The model under review builds one solid part; all positions refer to its coordinate system, in mm. A direction names the side the tool comes from. Round coordinates to 2 decimals unless told otherwise and drop trailing zeros. Order: outer loops, then holes, each group sorted by start corner. A loop starts at its lowest first (then second) coordinate and runs counter-clockwise, first axis right, second up.
from build123d import *

# Parameters (mm, degrees)
F0_W     = 127
F0_H     = 101.6
F1_DEPTH = 254
F2_SIZE  = 38.1
F3_W     = 50.8
F3_H     = 254
F4_DEPTH = 38.1
F5_SIZE  = 25.39999


# Not quite as in the source:
# - a fillet or chamfer is up to 0.001 mm smaller than in the source, because OpenCascade refuses the exact size


with BuildPart() as f1:
    # F0 (on Front) → F1 (new body)
    with BuildSketch(Plane.XZ):
        with Locations((63.5, 50.8)):
            Rectangle(F0_W, F0_H)
    extrude(amount=F1_DEPTH)

    # F2
    f2_edges = [f1.edges().sort_by_distance(p)[0] for p in [
        (127, -127, 101.6),
        (0, -127, 101.6),
    ]]
    chamfer(f2_edges, length=F2_SIZE)

    # F3 (on face) → F4 (join)
    with BuildSketch(Plane.XY.offset(101.6)):
        with Locations((63.5, -127)):
            Rectangle(F3_W, F3_H)
    extrude(amount=F4_DEPTH)

    # F5 (size 25.4 in the source; OpenCascade refuses exactly that, so slightly less here)
    f5_edges = [f1.edges().sort_by_distance(p)[0] for p in [
        (38.1, -127, 139.7),
        (88.9, -127, 139.7),
    ]]
    chamfer(f5_edges, length=F5_SIZE)


solid = f1.part
(1) Tool access review of faces 1 (the flat face through (38.1, -129, 108)), 2 (the flat face through (63, -125, 0)), 3 (the flat face through (88.9, -129, 108)): name each direction out of +Z, -Z, +X, -X, +Y, -Y from which nothing blocks a thin tool from reaching the whole face with its end or side.
(2) We need section B-B (x = 13.5). Give the boundary of the cut face in (y, z), and give its area (3 significant figures).
(3) Clearance check with flat-ended pins moving along their axes: P1, Ø5, axis at y = -109.5, z = 84.5, coming from the +X side; P2, Ø6, axis at x = 103.5, y = -132, coming from the +Z side; P3, Ø4, axis at y = -98, z = 114, coming from the +X side. State where each tip first meets the part, or that it passes through.
(4) To check wall thickness, follow L1, parallel to X at y = -172, z = 109; L2, parallel to X at y = -114, z = 131.5; L3, parallel to Z at x = 61, y = -84. State the ranges of each line that lie inside material, in increasing order.
(5) We need section C-C (z = 68.5). Give the boundary of the cut face in (x, y), and give its area (3 significant figures).
Verdict:
1. face 1: +Z, -X, +Y, -Y
1. face 2: -Z, +X, -X, +Y, -Y
1. face 3: +Z, +X, +Y, -Y
2. outline: (-254, 0) - (0, 0) - (0, 77) - (-254, 77) - close
2. area: 19,600 mm2
3. P1: stops at x = 108.5
3. P2: stops at z = 90
3. P3: stops at x = 88.9
4. L1: x = 38.1 to 88.9
4. L2: x = 55.3 to 71.7
4. L3: z = 0 to 137.2
5. outline: (5, -254) - (122, -254) - (122, 0) - (5, 0) - close
5. area: 29,700 mm2
